```python
from build123d import *

# Parameters (mm, degrees)
BASPROSKE_W     = 304.8
BASPROSKE_H     = 685.8
TOOTHCUT_DEPTH  = 1017.634801686
TEETHCUTS_COUNT = 25
TEETHCUTS_ANGLE = 345.6
BORSKE_R        = 127
BORE_DEPTH      = 304.8000508
KEYSKE_W        = 63.5
KEYSKE_H        = 154.8384
KEYWAY_DEPTH    = 304.8000508


with BuildPart() as part:
    # BasProSke → Base-Revolve (revolve)
    with BuildSketch(Plane(origin=(0, 0, 0), x_dir=(1, 0, 0), z_dir=(0, 1, 0)), mode=Mode.PRIVATE) as base_revolve_sk:
        with Locations((152.4, 342.9)):
            Rectangle(BASPROSKE_W, BASPROSKE_H)
    revolve(base_revolve_sk.sketch.rotate(Axis((-10, 0, 0), (1, 0, 0)), 180), axis=Axis((-10, 0, 0), (1, 0, 0)))

    # TooCutSke → ToothCut (cut, through all)
    with BuildSketch(Plane(origin=(0, 0, 0), x_dir=(0, 0, -1), z_dir=(1, 0, 0))):
        with BuildLine():
            ThreePointArc((28.961853932, 570.764407973), (0, 571.49873), (-28.961853932, 570.764407973))
            ThreePointArc((-28.961853932, 570.764407973), (-41.564862504, 628.900535379), (-67.343982953, 682.511001556))
            ThreePointArc((-67.343982953, 682.511001556), (0, 685.8254), (67.343982953, 682.511001556))
            ThreePointArc((67.343982953, 682.511001556), (41.564862504, 628.900535379), (28.961853932, 570.764407973))
        make_face()
    toothcut = extrude(amount=TOOTHCUT_DEPTH, mode=Mode.SUBTRACT)

    # TeethCuts: ToothCut ×25 about axis
    teethcuts_axis = Axis((-10, 0, 0), (1, 0, 0))
    for i in range(1, TEETHCUTS_COUNT):
        add(toothcut.rotate(teethcuts_axis, i * TEETHCUTS_ANGLE / (TEETHCUTS_COUNT - 1)), mode=Mode.SUBTRACT)

    # BorSke → Bore (cut, symmetric)
    with BuildSketch(Plane(origin=(0, 0, 0), x_dir=(0, 0, -1), z_dir=(1, 0, 0))):
        with Locations(Location((0, 0, 0), (0, 0, 180))):
            Circle(BORSKE_R)
    extrude(amount=BORE_DEPTH, both=True, mode=Mode.SUBTRACT)

    # KeySke → Keyway (cut, symmetric)
    with BuildSketch(Plane(origin=(0, 0, 0), x_dir=(0, 0, -1), z_dir=(1, 0, 0))):
        with Locations((0, 77.4192)):
            Rectangle(KEYSKE_W, KEYSKE_H)
    extrude(amount=KEYWAY_DEPTH, both=True, mode=Mode.SUBTRACT)


solid = part.part
```
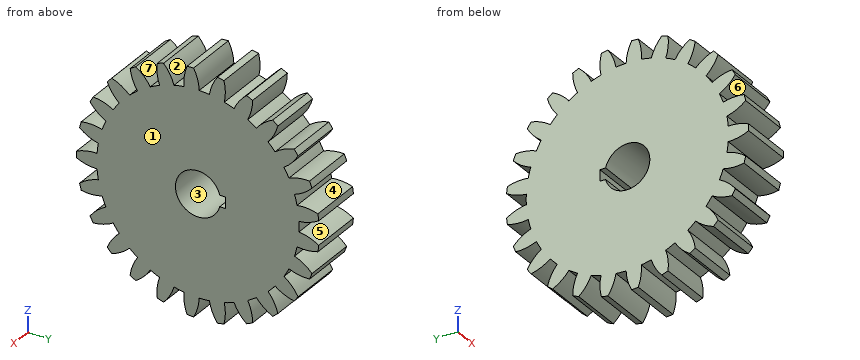
Design review of the part built by this model. Coordinates are the model's own, in mm. Face numbers are marked on the shaded views. A direction names the side the tool comes from. Round coordinates to 2 decimals unless told otherwise and drop trailing zeros. Order: outer loops, then holes, each group sorted by start corner. A loop starts at its lowest first (then second) coordinate and runs counter-clockwise, first axis right, second up. Notation, with made-up numbers: (21.25, -35.75) - (74.25, -35.75) arc R30 ccw to (74.25, -6.75) - close; hole circle Ø10 at (45.5, 21). An arc over 180 degrees is marked (long way). Return JSON: item names as keys, results as strings.
Q1. Consider section A-A on z = 0. Write out the cut boundary in (x, y), plus the area to 3 significant figures.
Computed values:
{"outline": "(0, -685.8) - (304.8, -685.8) - (304.8, -127) - (0, -127) - close; (0, 154.84) - (304.8, 154.84) - (304.8, 571.5) - (0, 571.5) - close", "area": "297,000 mm2"}
Q2. Machinability: for the marked faces 4, 5, 6 and 7, which of the approach directions +Z, -Z, +X, -X, +Y, -Y give a long, thin tool a straight path to every point of the face, cutting with its end or side? Answer none if there is none.
Computed values:
{"face 4": "+X, -X", "face 5": "+X, -X, +Y", "face 6": "+X, -X, -Y", "face 7": "+Z, +X, -X"}
Q3. For pin 1 Ø1.5 at (y, z) = (-169.5, -13) entering from -X; pin 2 Ø8 at (x, z) = (232.5, -495) entering from -Y; pin 3 Ø1 at (x, y) = (217.5, -412.5) entering from -Z; pin 4 Ø1 at (x, z) = (261, 496.5) entering from -Y, all flat-tipped, find the tip position at first contact; note any pin that passes through.
Computed values:
{"pin 1": "stops at x = 0", "pin 2": "stops at y = -363.95", "pin 3": "stops at z = -444.58", "pin 4": "stops at y = -363.06"}
Q4. The part is to be moulded in two halves that separate along Z. For the marked faces 1, 2 and 3, say which applies: pulls with the +Z half, pulls with the -Z half, needs draft (parallel to the pull), parting line crosses it, or undercut.
Computed values:
{"face 1": "needs draft", "face 2": "pulls with the +Z half", "face 3": "undercut"}
Q5. Wall thickness on L1, parallel to Y at x = 228, z = 0; L2, parallel to Y at x = 60, z = 508; L3, parallel to Y at x = 278, z = -619: over which ranges is each line inside the solid? List them lowest first. Write a range as [from, to].
Computed values:
{"L1": "y = [-685.8, -127], [154.84, 571.5]", "L2": "y = [-367.67, -271.58], [-261.81, 286.43], [371.17, 449.15]", "L3": "y = [-231.63, -164.09], [-77.87, 0.83], [78.55, 154.55], [264.33, 295.23]"}
